Check sheet for the modelled part. Datum: model origin and axes. Units: mm. Face numbers are marked on the shaded views. A direction names the side the tool comes from. Give positions to 0.01 mm unless a question says otherwise; leave off trailing zeros. Order: outer loops, then holes, each group sorted by start corner. A loop starts at its lowest first (then second) coordinate and runs counter-clockwise, first axis right, second up.
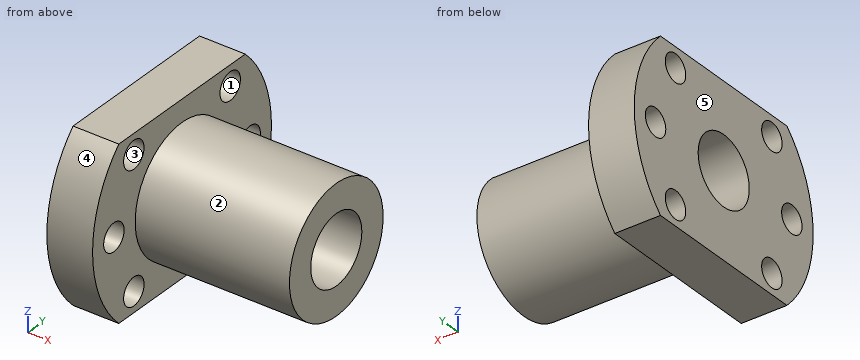
Autodesk Inventor part; units mm, degrees
ref_plane "YZ Plane" through (0, 0, 0) normal (1, 0, 0) x (0, 1, 0)
ref_plane "XZ Plane" through (0, 0, 0) normal (0, 1, 0) x (-1, 0, 0)
ref_plane "XY Plane" through (0, 0, 0) normal (0, 0, 1) x (1, 0, 0)
sketch "Sketch1" plane through (0, 0, 0) normal (0, 0, 1) x (1, 0, 0)
  line L0 (0, 21) -> (0, 6)
  line L1 (0, 0) -> (35, 0) construction
  line L2 (35, 0) -> (35, 6) construction
  line L3 (35, 11) -> (8, 11)
  line L4 (8, 11) -> (8, 21)
  line L5 (8, 21) -> (0, 21)
  line L6 (35, 6) -> (0, 6)
  line L7 (0, 6) -> (0, 0) construction
  line L8 (35, 6) -> (35, 11)
  dimension "d0" = 11
  dimension "d1" = 21
  dimension "d2" = 8
  dimension "d3" = 35
  dimension "d4" = 6
revolve "Revolution1" add sketch "Sketch1" angle 360 about axis through (0, 0, 0) along (1, 0, 0)
sketch "Sketch2" plane through (0, 0, 0) normal (-1, 0, 0) x (0, 0, 1)
  circle A0 centre (0, 0) radius 21
  circle A1 centre (0, 0) radius 21
  line L0 (-14.8492, 14.8492) -> (-14.8492, -14.8492)
  line L1 (14.8492, -14.8492) -> (14.8492, 14.8492)
  line L2 (0, 0) -> (14.8492, 14.8492) construction
  circle A2 centre (0, 16) radius 2.4
  circle A3 centre (11.3137, 11.3137) radius 2.4
  circle A4 centre (11.3137, -11.3137) radius 2.4
  circle A5 centre (0, 0) radius 16 construction
  circle A6 centre (-11.3137, 11.3137) radius 2.4
  circle A7 centre (0, -16) radius 2.4
  circle A8 centre (-11.3137, -11.3137) radius 2.4
  point P0 (-14.8492, -14.8492)
  dimension "d6" = 45
  dimension "d7" = 32
  dimension "d8" = 4.8
extrude "Extrusion1" cut sketch "Sketch2" against normal blind 10 contours A0 L1 | L0 A0 | A2 | A3 | A4 | A6 | A7 | A8
properties part number "SFU1204-Housing"
Q1. Sectioned sample at A-A, the plane z = 0. Record the cut outline in (x, y).
Q2. Sectioned sample at D-D, the plane x = 4. Record the cut outline in (y, z).
Q3. Go/stop test with flat-tipped pins: P1, Ø1, axis at y = -4.5, z = 6.5, coming from the -X side; P2, Ø2, axis at x = 6, z = -10.5, coming from the +Y side; P3, Ø1.5, axis at x = 7.5, z = 4.5, coming from the +Y side; P4, Ø4, axis at y = 11.31, z = 11.31, coming from the +X side. Record where each tip stops, or that it passes through.
Q4. Sectioned sample at B-B, the plane y = 16. Record the cut outline in (x, z).
Q5. Material ranges on line 1 (X direction, y = -13, z = 9.25); line 2 (Y direction, x = 24, z = -2.5); line 3 (Z direction, x = 33.5, y = 1), recorded low to high.
Q6. Tool access check on the marked faces 1 and 2. Record the directions out of +Z, -Z, +X, -X, +Y, -Y that give a thin tool (end or side, any length) a straight path to the whole face; none if there is none.
Q7. Sectioned sample at C-C, the plane z = -10. Record the cut outline in (x, y).
Q8. Draft check along Z on the marked faces 3, 4 and 5. Enter one of: pulls with the +Z half, pulls with the -Z half, needs draft (parallel to the pull), parting line crosses it, or undercut.
Filled in:
1. outline: (0, -21) - (8, -21) - (8, -18.4) - (0, -18.4) - close; (0, -13.6) - (8, -13.6) - (8, -11) - (35, -11) - (35, -6) - (0, -6) - close; (0, 6) - (35, 6) - (35, 11) - (8, 11) - (8, 13.6) - (0, 13.6) - close; (0, 18.4) - (8, 18.4) - (8, 21) - (0, 21) - close
2. outline: (-14.85, -14.85) - (14.85, -14.85) arc R21 ccw to (14.85, 14.85) - (-14.85, 14.85) arc R21 ccw to start; hole circle Ø4.8 at (-16, 0); hole circle Ø4.8 at (-11.31, -11.31); hole circle Ø4.8 at (-11.31, 11.31); hole circle Ø12 at (0, 0); hole circle Ø4.8 at (11.31, -11.31); hole circle Ø4.8 at (11.31, 11.31); hole circle Ø4.8 at (16, 0)
3. P1: stops at x = 0
3. P2: stops at y = 18.73
3. P3: stops at y = 20.66
3. P4: passes through
4. outline: (0, -13.6) - (8, -13.6) - (8, -2.4) - (0, -2.4) - close; (0, 2.4) - (8, 2.4) - (8, 13.6) - (0, 13.6) - close
5. line 1: x = 0 to 8
5. line 2: y = -10.71 to -5.45, 5.45 to 10.71
5. line 3: z = -10.95 to -5.92, 5.92 to 10.95
6. face 1: +X, -X
6. face 2: +X
7. outline: (0, -18.47) - (8, -18.47) - (8, -13.32) - (0, -13.32) - close; (0, -9.31) - (8, -9.31) - (8, -4.58) - (35, -4.58) - (35, 4.58) - (8, 4.58) - (8, 9.31) - (0, 9.31) - close; (0, 13.32) - (8, 13.32) - (8, 18.47) - (0, 18.47) - close
8. face 3: undercut
8. face 4: parting line crosses it
8. face 5: needs draft
